The listing builds one solid part. Answer for the finished solid, in the listing's coordinates (mm). Round coordinates to 2 decimals unless told otherwise and drop trailing zeros. Loops run counter-clockwise (first coordinate to the right, second up) from the corner with the lowest first, then second, coordinate; pieces in that order, holes last. Notation, with made-up numbers: (-5, 2.5) -> (30, 2.5) arc R10 ccw to (30, 11.5) -> close; hole circle Ø5 at (65.25, 43). An arc over 180 degrees is marked (long way). Write each question's results on one line, items separated by ' | '. Start each with the question number.
(1) The part is cut by section A-A (z = -3). Determine the outline of the cut face in (x, y).
(2) Flat-ended cylindrical pins translate along their axes: pin 1 (4 mm diameter, centred on y = 0.5, z = -1, fed in from -X); pin 2 (0.7 mm diameter, centred on y = -1.5, z = -3, fed in from -X); pin 3 (2 mm diameter, centred on x = 0.5, z = 0.5, fed in from -Y); pin 4 (0.6 mm diameter, centred on x = 1.5, y = -0.5, fed in from +Z). Find the tip coordinate at first contact, or state that the pin passes through.
(3) Straight lines are drawn through the part: probe 1 along Z at (x, y) = (1.25, -1); probe 2 along Y at (x, z) = (-1.75, 0); probe 3 along Y at (x, z) = (1.1, -4). For each, find the intervals that lie inside material, in ascending order.
(4) The part is cut by section B-B (x = 0). Determine the outline of the cut face in (y, z).
(5) The part is cut by section C-C (y = 2.75). Determine the outline of the cut face in (x, z).
(6) The part is cut by section D-D (x = -0.8). Determine the outline of the cut face in (y, z).
```python
from build123d import *

# Parameters (mm, degrees)
SKETCH2_W          = 0.45
SKETCH2_H          = 2.491987158
CUT_EXTRUDE1_DEPTH = 6.97452927
SKETCH3_W          = 0.5
SKETCH3_H          = 0.5


with BuildPart() as part:
    # Sketch1 → Revolve1 (revolve)
    with BuildSketch(Plane(origin=(0, 0, 0), x_dir=(1, 0, 0), z_dir=(0, 0, -1))):
        with BuildLine():
            Line((0, 0), (0, -5.3))
            ThreePointArc((0, -5.3), (1.060660172, -4.860660172), (1.5, -3.8))
            Line((1.5, -3.8), (1.5, -0.8))
            Line((1.5, -0.8), (1.95, -0.8))
            Line((1.95, -0.8), (1.95, 0))
            Line((1.95, 0), (0, 0))
        make_face()
    revolve(axis=Axis((0, 0, 0), (0, 1, 0)))

    # Sketch2 → Cut-Extrude1 (cut, through all)
    with BuildSketch(Plane(origin=(0, 0, 0), x_dir=(-1, 0, 0), z_dir=(0, -1, 0))):
        with Locations((-1.725, 0)):
            Rectangle(SKETCH2_W, SKETCH2_H)
    extrude(amount=-CUT_EXTRUDE1_DEPTH, mode=Mode.SUBTRACT)

    # Sweep1: sweep along a path in Sketch4
    with BuildLine(Plane(origin=(-1.27, 0, 0), x_dir=(0, 0, -1), z_dir=(1, 0, 0))) as sweep1_path:
        Line((0, 0), (0, -1))
        ThreePointArc((0, -1), (0.292893219, -1.707106781), (1, -2))
        Line((1, -2), (5, -2))
    # Sketch3 → Sweep1 (sweep)
    with BuildSketch(Plane(origin=(0, 0, 0), x_dir=(-1, 0, 0), z_dir=(0, -1, 0))):
        with Locations((-1.27, 0)):
            Rectangle(SKETCH3_W, SKETCH3_H)
        with Locations((1.27, 0)):
            Rectangle(SKETCH3_W, SKETCH3_H)
    sweep(path=sweep1_path.line)


solid = part.part
```
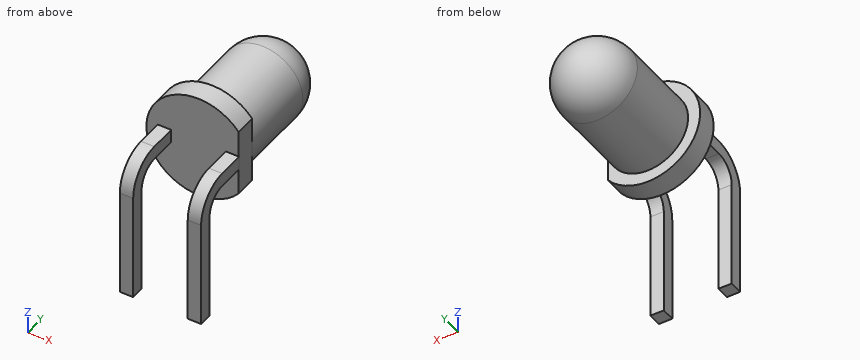
Checked values:
1) outline: (-1.52, -2.25) -> (-1.02, -2.25) -> (-1.02, -1.75) -> (-1.52, -1.75) -> close; (1.02, -2.25) -> (1.52, -2.25) -> (1.52, -1.75) -> (1.02, -1.75) -> close
2) pin 1: stops at x = -1.95 | pin 2: stops at x = -1.52 | pin 3: stops at y = -2.07 | pin 4: stops at z = 0.25
3) probe 1: z = -0.25 to 0.25 | probe 2: y = 0 to 0.8 | probe 3: y = -2.25 to -1.75
4) outline: (0, -1.95) -> (0.8, -1.95) -> (0.8, -1.5) -> (3.8, -1.5) arc R1.5 ccw to (3.8, 1.5) -> (0.8, 1.5) -> (0.8, 1.95) -> (0, 1.95) -> close
5) outline: circle Ø3 at (0, 0)
6) outline: (0, -1.78) -> (0.8, -1.78) -> (0.8, -1.27) -> (3.8, -1.27) arc R1.27 ccw to (3.8, 1.27) -> (0.8, 1.27) -> (0.8, 1.78) -> (0, 1.78) -> close
